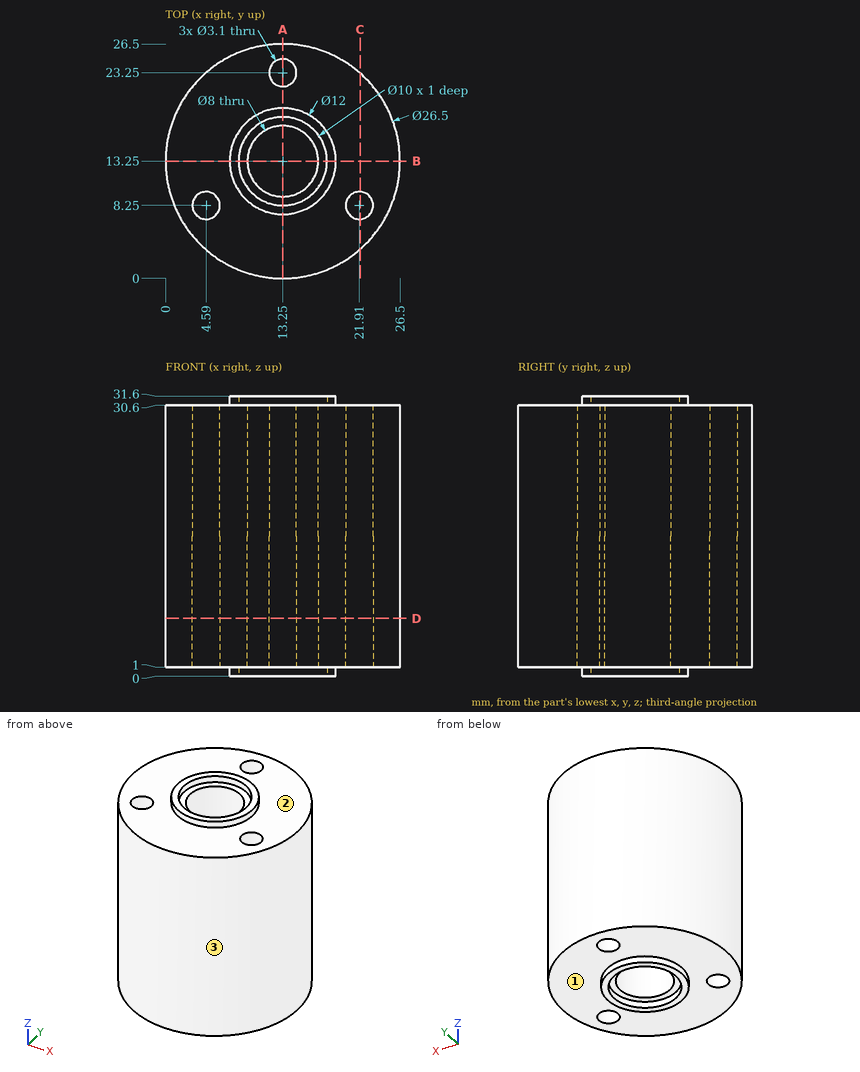
Drawing for the job (mm, zero at the part's lowest x, y, z). A direction names the side the tool comes from. Give positions to 0.01 mm unless a question says otherwise; leave off trailing zeros. Write each loop counter-clockwise with the first axis right and the second up, starting at its lowest first coordinate (ties: lowest second). Pieces come first, ordered by that corner, then holes. Notation, with made-up numbers: M 89.25,68 L 101.25,68 A15 cw 101.25,75 Z; hole C 53.5,53.5 d3. An arc over 180 degrees is marked long. Return JSON: item names as keys, results as strings. Group by question number.
(1) Band-saw the part on D-D (z = 6.5). Give the cut face in (x, y), and give its area (3 significant figures).
(2) Band-saw the part on A-A (x = 13.25). Give the cut face in (y, z).
(3) Band-saw the part on C-C (x = 22). Give the cut face in (y, z).
(4) Flat gauge pins, fed straight in: pin 1 Ø3 at (y, z) = (7.5, 21.5) entering from +X; pin 2 Ø10 at (x, y) = (20.5, 17.5) entering from -Z; pin 3 Ø12 at (y, z) = (22.5, 18) entering from +X (1 decimal); pin 4 Ø5 at (x, z) = (19.5, 18.5) entering from -Y. Where does each tip first touch, or does it go through?
(5) Drill centre lines: L1, parallel to Y at x = 13.25, z = 25.5; L2, parallel to Y at x = 13.25, z = 0.7; L3, parallel to Y at x = 13.75, z = 29.5. Where is each one in solid material? Low to high. Write a range as [from, to].
(6) 3-axis set-ups, long thin cutter, end or side, ignore diameter. For the marked faces 1, 2 and 3: which of +Z, -Z, +X, -X, +Y, -Y reach the whole face in a straight line?
(7) Band-saw the part on B-B (y = 13.25). Give the cut face in (x, z).
Entries:
{
 "1": {"outline": "C 13.25,13.25 d26.5; hole C 4.59,8.25 d3.1; hole C 13.25,13.25 d8; hole C 13.25,23.25 d3.1; hole C 21.91,8.25 d3.1", "area": "479 mm^2"},
 "2": {"outline": "M 0,1 L 7.25,1 L 7.25,0 L 8.25,0 L 8.25,1 L 9.25,1 L 9.25,30.6 L 8.25,30.6 L 8.25,31.6 L 7.25,31.6 L 7.25,30.6 L 0,30.6 Z; M 17.25,1 L 18.25,1 L 18.25,0 L 19.25,0 L 19.25,1 L 21.7,1 L 21.7,30.6 L 19.25,30.6 L 19.25,31.6 L 18.25,31.6 L 18.25,30.6 L 17.25,30.6 Z; M 24.8,1 L 26.5,1 L 26.5,30.6 L 24.8,30.6 Z"},
 "3": {"outline": "M 3.3,1 L 6.7,1 L 6.7,30.6 L 3.3,30.6 Z; M 9.8,1 L 23.2,1 L 23.2,30.6 L 9.8,30.6 Z"},
 "4": {"pin 1": "stops at x = 25.8", "pin 2": "stops at z = 0", "pin 3": "stops at x = 26.1", "pin 4": "stops at y = 0.54"},
 "5": {"L1": "y = [0, 9.25], [17.25, 21.7], [24.8, 26.5]", "L2": "y = [7.25, 8.25], [18.25, 19.25]", "L3": "y = [0.01, 9.28], [17.22, 21.78], [24.72, 26.49]"},
 "6": {"face 1": "-Z", "face 2": "+Z", "face 3": "+Z, -Z"},
 "7": {"outline": "M 0,1 L 7.25,1 L 7.25,0 L 8.25,0 L 8.25,1 L 9.25,1 L 9.25,30.6 L 8.25,30.6 L 8.25,31.6 L 7.25,31.6 L 7.25,30.6 L 0,30.6 Z; M 17.25,1 L 18.25,1 L 18.25,0 L 19.25,0 L 19.25,1 L 26.5,1 L 26.5,30.6 L 19.25,30.6 L 19.25,31.6 L 18.25,31.6 L 18.25,30.6 L 17.25,30.6 Z"}
}
